Here's how the part is built. I have some questions about the finished solid (model axes, mm). A direction names the side the tool comes from. Round coordinates to 2 decimals unless told otherwise and drop trailing zeros. Order: outer loops, then holes, each group sorted by start corner. A loop starts at its lowest first (then second) coordinate and runs counter-clockwise, first axis right, second up. Notation, with made-up numbers: M 45,6 L 50,6 A38 ccw 50,44 Z; hole C -30.75,68 d7. An arc over 180 degrees is marked long. Write each question's results on one line, items separated by ' | '. Start each with the question number.
```python
from build123d import *

# Parameters (mm, degrees)
SKETCH_2_R                   = 60
EXTRUDE_1_DEPTH              = 14
HOLE_WIZARD_M6_1_D           = 6.6
HOLE_WIZARD_M6_1_CBORE_D     = 11
HOLE_WIZARD_M6_1_CBORE_DEPTH = 6
PATTERN_CIRCULAR_1_COUNT     = 6
HOLE_WIZARD_M4_1_D           = 4.5
HOLE_WIZARD_M4_1_CBORE_D     = 8
HOLE_WIZARD_M4_1_CBORE_DEPTH = 4
SKETCH_9_R                   = 25
CUT_EXTRUDE_1_DEPTH          = 15


with BuildPart() as part:
    # 草圖2 → 填料-伸長1 (new body)
    with BuildSketch(Plane.XY):
        with Locations((0, -84)):
            Circle(SKETCH_2_R)
    extrude(amount=EXTRUDE_1_DEPTH)

    # M6 承窩頭蓋螺釘的柱孔1 (through all)
    with Locations(Plane.XY.offset(14)):
        with Locations((52.159798329, -89.96702927)):
            hole_wizard_m6_1 = CounterBoreHole(HOLE_WIZARD_M6_1_D / 2, HOLE_WIZARD_M6_1_CBORE_D / 2, HOLE_WIZARD_M6_1_CBORE_DEPTH)

    # 環狀複製排列1: M6 承窩頭蓋螺釘的柱孔1 ×6 about axis
    pattern_circular_1_axis = Axis((0, -84, 0), (0, 0, 1))
    for i in range(1, PATTERN_CIRCULAR_1_COUNT):
        add(hole_wizard_m6_1.rotate(pattern_circular_1_axis, i * 360 / PATTERN_CIRCULAR_1_COUNT), mode=Mode.SUBTRACT)

    # M4 承窩頭蓋螺釘的柱孔1 (through all)
    with Locations(Plane(origin=(0, 0, 0), x_dir=(-1, 0, 0), z_dir=(0, 0, -1))):
        with Locations((0, -53), (-11.863186403, -55.359734492), (-21.920310217, -62.079689783), (-28.640265508, -72.136813597), (-31, -84), (-28.640265508, -95.863186403), (-21.920310217, -105.920310217), (-11.863186403, -112.640265508), (0, -115), (11.863186403, -112.640265508), (21.920310217, -105.920310217), (28.640265508, -95.863186403), (31, -84), (28.640265508, -72.136813597), (21.920310217, -62.079689783), (11.863186403, -55.359734492)):
            CounterBoreHole(HOLE_WIZARD_M4_1_D / 2, HOLE_WIZARD_M4_1_CBORE_D / 2, HOLE_WIZARD_M4_1_CBORE_DEPTH)

    # 草圖9 → 除料-伸長1 (cut, through all)
    with BuildSketch(Plane.XY.offset(14)):
        with Locations((0, -84)):
            Circle(SKETCH_9_R)
    extrude(amount=-CUT_EXTRUDE_1_DEPTH, mode=Mode.SUBTRACT)


solid = part.part
```
(1) If we mould it in two halves opening along X, with no side actions, what happens to faces 4 (the flat face through (-55, -76, 8)), 5 (the flat face through (26, -83, 0))? For each: pulls with the +X half, pulls with the -X half, needs draft (parallel to the pull), parting line crosses it, or undercut.
(2) I want a section at C-C on x = 40. Write out the boundary of the cut face in (y, z), and give its area (3 significant figures).
(3) On a 3-axis mill with a long thin cutter (end or side, diameter ignored), from which of +Z, -Z, +X, -X, +Y, -Y can I reach the whole of each face in a straight line? I mean faces 1 (the cylindrical face through (-13.71, -116.19, 1.97)), 2 (the cylindrical face through (20.26, -60.56, 9.07)), 3 (the cylindrical face through (-54.698, -73.154, 11.042)). Say none if no direction works.
(4) Please list where these lines run through material, in increasing order: line 1 (X direction, y = -83.5, z = 3.25) (3 decimals); line 2 (X direction, y = -96, z = 1.5); line 3 (X direction, y = -92.5, z = 4.25) (3 decimals).
(5) I'm going to push flat-ended pins straight in: pin 1 Ø4 at (y, z) = (-48, 3.5) entering from -X; pin 2 Ø1 at (y, z) = (-113.5, 4) entering from -X; pin 3 Ø4 at (x, y) = (-30.5, -84.5) entering from -Z. Where does each tip first touch, or does it pass through?
(6) I want a section at B-B on z = 9.5. Give the number of separate pieces and of enclosed holes in the cut face, and give its area (3 significant figures).
(7) I want a section at A-A on x = -52.5. Write out the boundary of the cut face in (y, z).
Solutions:
1) face 4: undercut | face 5: needs draft
2) outline: M -128.72,0 L -39.28,0 L -39.28,14 L -128.72,14 Z | area: 1,250 mm^2
3) face 1: -Z | face 2: +Z, -Z | face 3: +Z
4) line 1: -59.998 to -34.969, -27.031 to -24.995, 24.995 to 27.031, 34.969 to 59.998 | line 2: -58.79 to -32.64, -24.64 to -21.93, 21.93 to 24.64, 32.64 to 58.79 | line 3: -59.395 to -23.511, 23.511 to 50.045, 54.275 to 59.395
5) pin 1: x = -49.44 | pin 2: x = -52.53 | pin 3: z = 4
6) separate pieces: 1 | enclosed holes: 23 | area: 8,520 mm^2
7) outline: M -113.05,0 L -81.32,0 L -81.32,8 L -83.52,8 L -83.52,14 L -113.05,14 Z; M -74.75,0 L -54.95,0 L -54.95,14 L -72.54,14 L -72.54,8 L -74.75,8 Z
